The listing builds one solid part. Answer for the finished solid, in the listing's coordinates (mm). A direction names the side the tool comes from. Coordinates: 2 decimals unless noted, no trailing zeros. Order: outer loops, then holes, each group sorted by start corner. A loop starts at its lowest first (then second) coordinate and runs counter-clockwise, first axis right, second up. Notation, with made-up numbers: (-33.5, 51) -> (10.5, 51) arc R19 cw to (10.5, 72) -> close; hole circle Ø8 at (36.25, 7.5). An arc over 180 degrees is marked (long way). Return JSON: item names as keys, results as strings.
from build123d import *

# Parameters (mm, degrees)
SKETCH1_R           = 16
SKETCH1_R_2         = 11
BOSS_EXTRUDE1_DEPTH = 11
BOSS_EXTRUDE2_DEPTH = 17.5
BOSS_EXTRUDE3_DEPTH = 7.5
CHAMFER1_SIZE       = 1.5
FILLET1_RADIUS      = 7.5
FILLET1_LENGTH      = 22
FILLET2_RADIUS      = 7.5
FILLET2_LENGTH      = 22
SKETCH2_R           = 5
CUT_EXTRUDE1_DEPTH  = 202.748605943


with BuildPart() as part:
    # Sketch1 → Boss-Extrude1 (new, symmetric)
    with BuildSketch(Plane(origin=(0, 0, 0), x_dir=(1, 0, 0), z_dir=(0, 1, 0))):
        with Locations(Location((180, 0, 0), (0, 0, 270))):
            Circle(SKETCH1_R)
        with Locations(Location((180, 0, 0), (0, 0, 270))):
            Circle(SKETCH1_R_2, mode=Mode.SUBTRACT)
    extrude(amount=BOSS_EXTRUDE1_DEPTH, both=True)



with BuildPart() as body_2:
    # Sketch1<3> → Boss-Extrude2 (new, symmetric)
    with BuildSketch(Plane(origin=(0, 0, 0), x_dir=(1, 0, 0), z_dir=(0, 1, 0))):
        with BuildLine():
            Line((0, 31), (0, 25))
            ThreePointArc((0, 25), (25, 0), (0, -25))
            Line((0, -25), (0, -31))
            ThreePointArc((0, -31), (31, 0), (0, 31))
        make_face()
    extrude(amount=BOSS_EXTRUDE2_DEPTH, both=True)


with BuildPart() as part_1:
    add(part.part)

    add(body_2.part)  # Boss-Extrude3 merges body 2
    # Sketch1<4> → Boss-Extrude3 (add, symmetric)
    with BuildSketch(Plane(origin=(0, 0, 0), x_dir=(1, 0, 0), z_dir=(0, 1, 0))):
        with BuildLine():
            Line((0, 44.5), (0, 31))
            ThreePointArc((0, 31), (31, 0), (0, -31))
            Line((0, -31), (0, -44.5))
            Line((0, -44.5), (22, -44.5))
            Line((22, -44.5), (22, -33.163866466))
            ThreePointArc((22, -33.163866466), (22.416915225, -31.165033321), (23.598133576, -29.499537764))
            ThreePointArc((23.598133576, -29.499537764), (38.131334863, -20.095927671), (55, -16.211348046))
            Line((55, -16.211348046), (154.726094768, -10.984924882))
            Line((154.726094768, -10.984924882), (160.111143378, -10.702706443))
            ThreePointArc((160.111143378, -10.702706443), (166.09109505, -11.293263792), (171.625716668, -13.633465395))
            ThreePointArc((171.625716668, -13.633465395), (164, 0), (171.625716668, 13.633465395))
            ThreePointArc((171.625716668, 13.633465395), (166.09109505, 11.293263792), (160.111143378, 10.702706443))
            Line((160.111143378, 10.702706443), (154.726094768, 10.984924882))
            Line((154.726094768, 10.984924882), (55, 16.211348046))
            ThreePointArc((55, 16.211348046), (38.131334863, 20.095927671), (23.598133576, 29.499537764))
            ThreePointArc((23.598133576, 29.499537764), (22.416915225, 31.165033321), (22, 33.163866466))
            Line((22, 33.163866466), (22, 44.5))
            Line((22, 44.5), (0, 44.5))
        make_face()
        with BuildLine():
            Line((54.738320219, 11.218200372), (154.464414987, 5.991777209))
            ThreePointArc((154.464414987, 5.991777209), (160.15039925, 0), (154.464414987, -5.991777209))
            Line((154.464414987, -5.991777209), (54.738320219, -11.218200372))
            ThreePointArc((54.738320219, -11.218200372), (42.916803625, 0), (54.738320219, 11.218200372))
        make_face(mode=Mode.SUBTRACT)
    extrude(amount=BOSS_EXTRUDE3_DEPTH, both=True)

    # Chamfer1
    chamfer1_edges = [part_1.edges().sort_by_distance(p)[0] for p in [
        (160.15039925, 7.5, 0),
        (104.601367603, -7.5, 8.60498879),
        (42.916803625, 7.5, 0),
        (104.601367603, 7.5, -8.60498879),
        (104.601367603, 7.5, 8.60498879),
        (160.15039925, -7.5, 0),
        (104.601367603, -7.5, -8.60498879),
        (42.916803625, -7.5, 0),
        (180, -11, -11),
        (180, 11, -11),
    ]]
    chamfer(chamfer1_edges, length=CHAMFER1_SIZE)

    # Fillet1: full round fillet: the end face becomes a half cylinder, R = half its width
    fillet1_face = Plane((11, 0, 44.5), x_dir=(1, 0, 0), z_dir=(0, 0, 1))  # on the end face: x along it, z out of the body
    fillet1_slab = fillet1_face.offset(-FILLET1_RADIUS / 2) * Box(FILLET1_LENGTH, 2 * FILLET1_RADIUS, FILLET1_RADIUS, mode=Mode.PRIVATE)  # the body's end, R deep
    fillet1_round = Plane((11, 0, 37), x_dir=(0, 0, 1), z_dir=(1, 0, 0)) * Cylinder(FILLET1_RADIUS, FILLET1_LENGTH, mode=Mode.PRIVATE)  # its axis R under the face
    add(fillet1_slab - fillet1_round, mode=Mode.SUBTRACT)

    # Fillet2: full round fillet: the end face becomes a half cylinder, R = half its width
    fillet2_face = Plane((11, 0, -44.5), x_dir=(1, 0, 0), z_dir=(0, 0, -1))  # on the end face: x along it, z out of the body
    fillet2_slab = fillet2_face.offset(-FILLET2_RADIUS / 2) * Box(FILLET2_LENGTH, 2 * FILLET2_RADIUS, FILLET2_RADIUS, mode=Mode.PRIVATE)  # the body's end, R deep
    fillet2_round = Plane((11, 0, -37), x_dir=(0, 0, -1), z_dir=(1, 0, 0)) * Cylinder(FILLET2_RADIUS, FILLET2_LENGTH, mode=Mode.PRIVATE)  # its axis R under the face
    add(fillet2_slab - fillet2_round, mode=Mode.SUBTRACT)

    # Sketch2 → Cut-Extrude1 (cut, through all)
    with BuildSketch(Plane.ZY):
        with Locations((-37, 0)):
            Circle(SKETCH2_R)
        with Locations((37, 0)):
            Circle(SKETCH2_R)
    extrude(amount=-CUT_EXTRUDE1_DEPTH, mode=Mode.SUBTRACT)


solid = part_1.part
1. Determine the mould class of faces 1 (the face through (11.15, 0.16, 44.5)), 2 (the face through (105.3, 0.08, 8.57)), 3 (the face through (11, 0, -42)) for opening direction Y: pulls with the +Y half, pulls with the -Y half, needs draft (parallel to the pull), parting line crosses it, or undercut.
Answer block:
{"face 1": "parting line crosses it", "face 2": "needs draft", "face 3": "undercut"}
2. The part is cut by section B-B on z = 0. Give the vertices of the cut face in (x, y).
Answer block:
{"outline": "(25, -17.5) -> (31, -17.5) -> (31, -7.5) -> (41.42, -7.5) -> (42.92, -6) -> (42.92, 6) -> (41.42, 7.5) -> (31, 7.5) -> (31, 17.5) -> (25, 17.5) -> close; (160.15, -6) -> (161.65, -7.5) -> (164, -7.5) -> (164, -11) -> (167.5, -11) -> (169, -9.5) -> (169, 9.5) -> (167.5, 11) -> (164, 11) -> (164, 7.5) -> (161.65, 7.5) -> (160.15, 6) -> close; (191, -9.5) -> (192.5, -11) -> (196, -11) -> (196, 11) -> (192.5, 11) -> (191, 9.5) -> close"}
3. Each of these flat-tipped pins is pushed along its axis until it touches: pin 1 Ø6 at (x, z) = (78, -14.5) entering from -Y; pin 2 Ø6 at (x, z) = (139.5, -5.5) entering from +Y; pin 3 Ø16 at (y, z) = (0, 37) entering from +X. Where does it stop, or does it pass through?
Answer block:
{"pin 1": "stops at y = -7.5", "pin 2": "stops at y = 7.5", "pin 3": "stops at x = 24.14"}
4. Consider line 1 (X direction, y = -3.25, z = 0); line 2 (Y direction, x = 17, z = -37); line 3 (Z direction, x = 59, y = 3). Determine where each line is inside the solid, lowest interval first. Write a range as from..to.
Answer block:
{"line 1": "x = 25..42.92, 160.15..169, 191..196", "line 2": "y = -7.5..-5, 5..7.5", "line 3": "z = -16..-10.99, 10.99..16"}
5. The part is cut by section A-A on x = 180. Give the vertices of the cut face in (y, z).
Answer block:
{"outline": "(-11, -16) -> (11, -16) -> (11, -12.5) -> (9.5, -11) -> (-9.5, -11) -> (-11, -12.5) -> close; (-11, 12.5) -> (-9.5, 11) -> (9.5, 11) -> (11, 12.5) -> (11, 16) -> (-11, 16) -> close"}
6. The part is cut by section D-D on x = 131.5. Give the vertices of the cut face in (y, z), and give its area (3 significant figures).
Answer block:
{"outline": "(-7.5, -12.2) -> (7.5, -12.2) -> (7.5, -8.7) -> (6, -7.2) -> (-6, -7.2) -> (-7.5, -8.7) -> close; (-7.5, 8.7) -> (-6, 7.2) -> (6, 7.2) -> (7.5, 8.7) -> (7.5, 12.2) -> (-7.5, 12.2) -> close", "area": "146 mm2"}
7. For faces 4 (the face through (160.39, 6.24, -0.13)), 5 (the face through (172, 11, -10)), 6 (the face through (172, -11, -10)), determine the directions among +Z, -Z, +X, -X, +Y, -Y from which every point of the face is accessible in a straight line to the end or side of a thin tool.
Answer block:
{"face 4": "+Y", "face 5": "+Z, -Z, +X, +Y", "face 6": "+Z, -Z, +X, -Y"}
8. The part is cut by section C-C on z = 18.5. Give the vertices of the cut face in (x, y), and give its area (3 significant figures).
Answer block:
{"outline": "(16.82, -17.5) -> (24.87, -17.5) -> (24.87, -7.5) -> (42.45, -7.5) -> (42.45, 7.5) -> (24.87, 7.5) -> (24.87, 17.5) -> (16.82, 17.5) -> close", "area": "546 mm2"}
